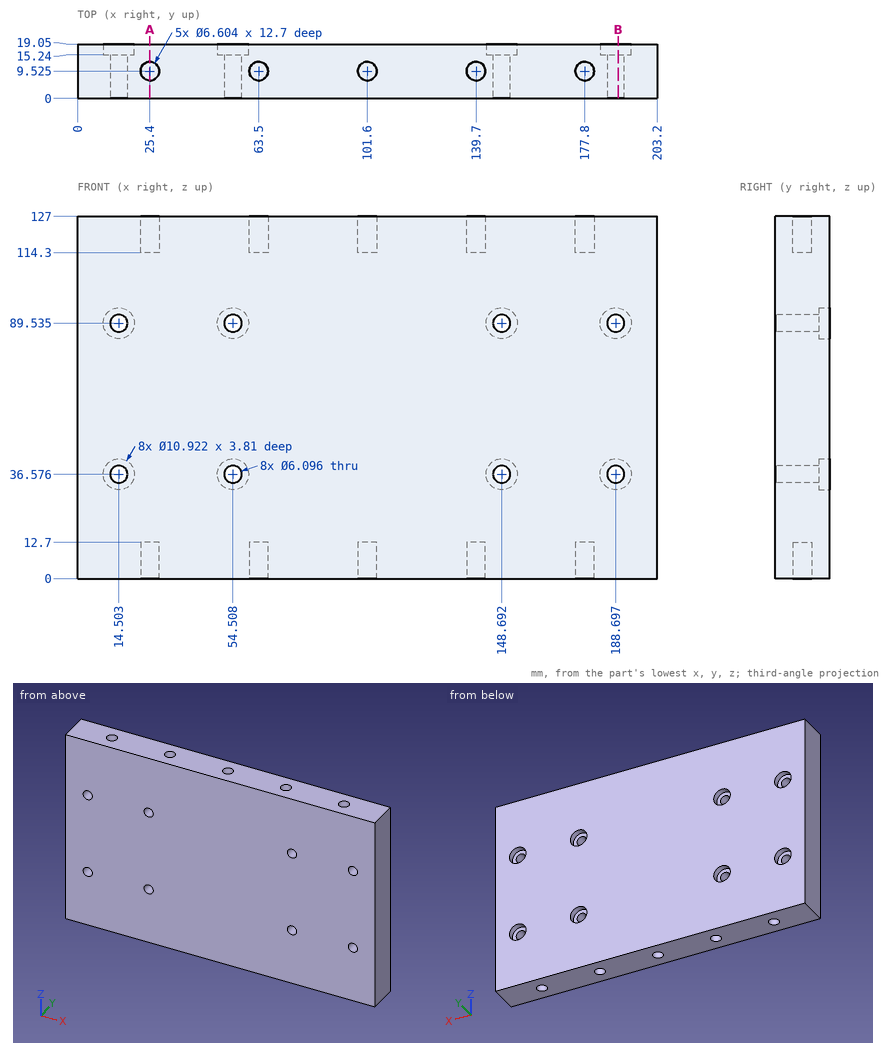
Part print with two shaded views. Sizes in mm from the minimum x, y, z corner. Round coordinates to 2 decimals unless told otherwise and drop trailing zeros. Order: outer loops, then holes, each group sorted by start corner. A loop starts at its lowest first (then second) coordinate and runs counter-clockwise, first axis right, second up. Notation, with made-up numbers: M 44,53 L 80,53 A37 ccw 80,89 Z; hole C -23,69 d1. An arc over 180 degrees is marked long. Put each result on its own line as item: value. Start each with the question number.
1. Slice it at A-A on x = 25.4. List the corners of the cut face in (y, z), then the cut area to 3 significant figures.
2. Drop flat-ended pins along their axis: pin 1 (4 mm diameter, centred on y = 17, z = 29.5, fed in from -X); pin 2 (4 mm diameter, centred on x = 63.5, y = 9.525, fed in from -Z); pin 3 (6.5 mm diameter, centred on x = 188.7, z = 89.54, fed in from +Y); pin 4 (5.5 mm diameter, centred on x = 177.8, y = 9.525, fed in from +Z). Give the stop position or say it passes through.
3. Slice it at B-B on x = 189.5. State how many separate pieces and enclosed holes the cut face has, then the cut area to 3 significant figures.
4. Drill centre lines: probe 1 along Z at (x, y) = (55, 12.75) (1 decimal); probe 2 along Y at (x, z) = (139.7, 119.5); probe 3 along Y at (x, z) = (16, 33). Where is each one in solid material? Low to high. Write a range as [from, to].
Findings:
1. outline: M 0,0 L 6.22,0 L 6.22,12.7 L 12.83,12.7 L 12.83,0 L 19.05,0 L 19.05,127 L 12.83,127 L 12.83,114.3 L 6.22,114.3 L 6.22,127 L 0,127 Z
1. area: 2,250 mm2
2. pin 1: x = 0
2. pin 2: z = 12.7
2. pin 3: y = 15.24
2. pin 4: z = 114.3
3. separate pieces: 3
3. enclosed holes: 0
3. area: 2,160 mm2
4. probe 1: [0, 33.6], [39.6, 86.5], [92.5, 127]
4. probe 2: [0, 6.22], [12.83, 19.05]
4. probe 3: [0, 15.24]
